Verification items for this drawing (mm, ordinates from the low corner). A direction names the side the tool comes from. Round coordinates to 2 decimals unless told otherwise and drop trailing zeros. Write each loop counter-clockwise with the first axis right and the second up, starting at its lowest first coordinate (ties: lowest second). Pieces come first, ordered by that corner, then holes. Notation, with made-up numbers: M 35,71 L 70,71 A18 cw 70,102 Z; hole C 75.5,37 d1. An arc over 180 degrees is marked long. One line per question, with ' | ' between items. Start each with the question number.
Q1. Cross-section at A-A (z = 6). Record the boundary of the cut face in (x, y), then the cut area to 3 significant figures.
Q2. Cross-section at C-C (x = 15). Record the boundary of the cut face in (y, z).
Q3. Thickness scan on line 1 along Y through (x, z) = (33.5, 27.5); line 2 along Z through (x, y) = (24.5, 1.5); line 3 along Y through (x, z) = (16.5, 30.5). Record the ranges inside material, lowest first. Write a range as from..to.
Q4. Tool access check on the marked faces 1 and 2. Record the directions out of +Z, -Z, +X, -X, +Y, -Y that give a thin tool (end or side, any length) a straight path to the whole face; none if there is none.
Q5. Gauge pin test, flat ends, axial feed: pin 1 (1.3 mm diameter, centred on y = 2, z = 11, fed in from -X); pin 2 (2 mm diameter, centred on x = 26, y = 1, fed in from +Z); pin 3 (3 mm diameter, centred on x = 35, y = 7.5, fed in from -Z); pin 4 (3 mm diameter, centred on x = 40, y = 2.5, fed in from +Z). Record the tip position at first contact, or that the pin passes through.
Q6. Cross-section at D-D (x = 36.5). Record the boundary of the cut face in (y, z), then the cut area to 4 significant figures.
Q7. Cross-section at B-B (y = 2.75). Record the boundary of the cut face in (x, z), then the cut area to 3 significant figures.
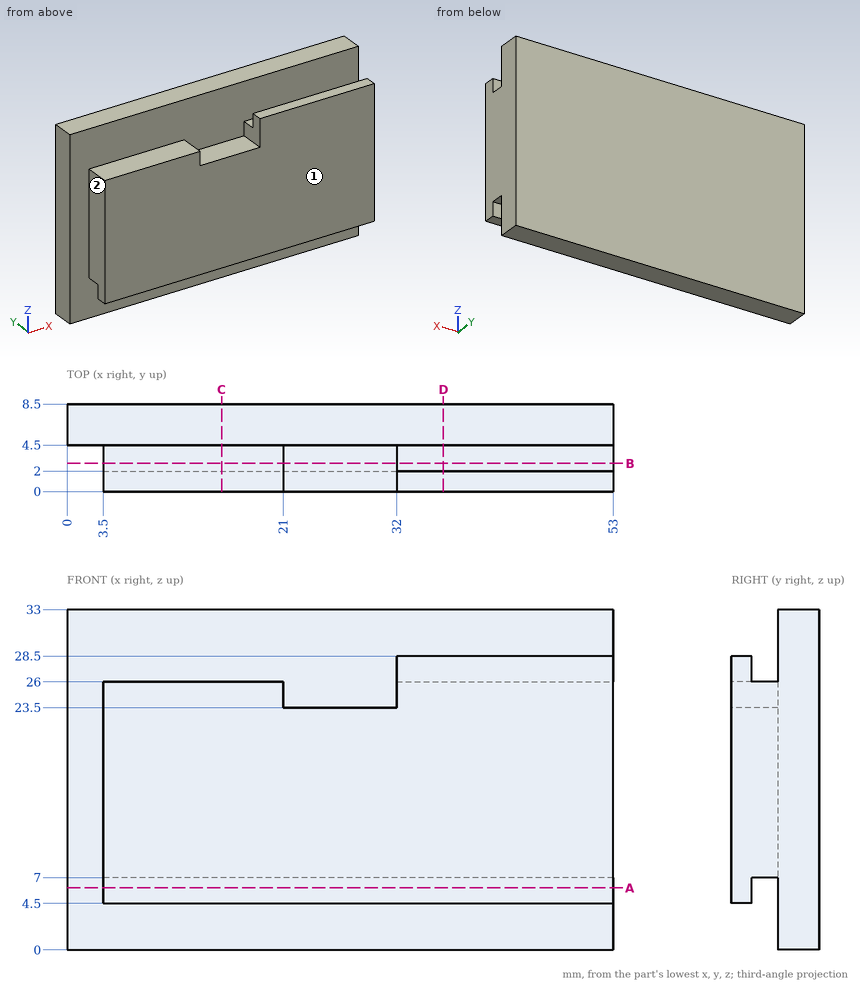
Determined:
1) outline: M 0,4.5 L 53,4.5 L 53,8.5 L 0,8.5 Z; M 3.5,0 L 53,0 L 53,2 L 3.5,2 Z | area: 311 mm²
2) outline: M 0,4.5 L 2,4.5 L 2,7 L 4.5,7 L 4.5,0 L 8.5,0 L 8.5,33 L 4.5,33 L 4.5,26 L 0,26 Z
3) line 1: y = 0..2, 4.5..8.5 | line 2: z = 4.5..23.5 | line 3: y = 4.5..8.5
4) face 1: +Z, -Z, +X, -X, -Y | face 2: +Z, -Z, -X, -Y
5) pin 1: stops at x = 3.5 | pin 2: stops at z = 23.5 | pin 3: stops at z = 0 | pin 4: stops at z = 28.5
6) outline: M 0,4.5 L 2,4.5 L 2,7 L 4.5,7 L 4.5,0 L 8.5,0 L 8.5,33 L 4.5,33 L 4.5,26 L 2,26 L 2,28.5 L 0,28.5 Z | area: 227.5 mm²
7) outline: M 3.5,7 L 53,7 L 53,26 L 32,26 L 32,23.5 L 21,23.5 L 21,26 L 3.5,26 Z | area: 913 mm²
